Geometry check sheet. Reference: the model listing, model coordinates, mm. Give positions to 0.01 mm unless a question says otherwise; leave off trailing zeros. Write each loop counter-clockwise with the first axis right and the second up, starting at its lowest first coordinate (ties: lowest second). Pieces come first, ordered by that corner, then holes. Notation, with made-up numbers: (-6, -17.75) - (51, -17.75) arc R10 cw to (51, -7.75) - close; hole circle Ø9 at (-15.75, 17). An arc over 180 degrees is marked (long way). Write item = value, one per line. Start each with the question number.
(1) Section check B-B, the plane z = -0.5. Enter the section's corners in (x, y), plus the area to 3 significant figures.
(2) Section check A-A, the plane x = 0. Enter the section's corners in (y, z), plus the area to 3 significant figures.
(3) Thickness scan on L1, parallel to X at y = -7, z = -1.5; L2, parallel to Y at x = -0.25, z = -0.5; L3, parallel to Z at x = 2, y = -6.75. Record the ranges inside material, lowest first.
(4) Section check C-C, the plane z = 10.5. Enter the section's corners in (x, y).
(5) Draft check along X on faces 1 (the cylindrical face through (0.41, -10.123, 28.602)), 2 (the flat face through (0, -4, -11)), 3 (the flat face through (0, -4.35, -5)), 4 (the flat face through (0, -7, 1)). Enter one of: pulls with the +X half, pulls with the -X half, needs draft (parallel to the pull), parting line crosses it, or undercut.
(6) Depth check by flat-ended pin: pin 1 Ø1.8 at (x, y) = (0.5, -7.5) entering from -Z; pin 2 Ø4 at (x, z) = (-1, 25.5) entering from +Y; pin 3 Ø1.5 at (y, z) = (-8.5, 9.5) entering from -X. Enter the tip coordinate at first touch or a pass-through.
```python
from build123d import *

# Parameters (mm, degrees)
BOSS_EXTRUDE1_DEPTH      = 1
BOSS_EXTRUDE1_DEPTH_BACK = 11
BOSS_EXTRUDE2_DEPTH      = 15
SKETCH3_R                = 3.15
BOSS_EXTRUDE3_DEPTH      = 21
FILLET1_R                = 12


with BuildPart() as part:
    # Sketch1 → Boss-Extrude1 (new, two sides: drawn at the far end of the back side and taken through both)
    with BuildSketch(Plane.XY.offset(-BOSS_EXTRUDE1_DEPTH_BACK)):
        with BuildLine():
            Line((2.107130751, -3.6), (-2.107130751, -3.6))
            ThreePointArc((-2.107130751, -3.6), (-3.494890771, -5.054302567), (-4, -7))
            ThreePointArc((-4, -7), (1.945697433, -10.494890771), (2.107130751, -3.6))
        make_face()
        with BuildLine():
            Line((1.881488772, -4.35), (-1.881488772, -4.35))
            ThreePointArc((-1.881488772, -4.35), (-2.887675407, -5.508748598), (-3.25, -7))
            ThreePointArc((-3.25, -7), (1.491251402, -9.887675407), (1.881488772, -4.35))
        make_face(mode=Mode.SUBTRACT)
    extrude(amount=BOSS_EXTRUDE1_DEPTH + BOSS_EXTRUDE1_DEPTH_BACK)

    # Sketch2 → Boss-Extrude2 (add)
    with BuildSketch(Plane.XY.offset(1)):
        with BuildLine():
            Line((2.107130751, -3.6), (-2.107130751, -3.6))
            ThreePointArc((-2.107130751, -3.6), (0, -11), (2.107130751, -3.6))
        make_face()
    extrude(amount=BOSS_EXTRUDE2_DEPTH)

    # Sketch3 → Boss-Extrude3 (add)
    with BuildSketch(Plane.XY.offset(16)):
        with Locations(Location((0, -7, 0), (0, 0, 180))):
            Circle(SKETCH3_R)
    extrude(amount=BOSS_EXTRUDE3_DEPTH)

    # Fillet1
    # the kernel refuses this fillet: 12 mm, written as the material it adds along each edge
    with BuildSketch(Plane(origin=(0, -7, 16), x_dir=(-1, 0, 0), z_dir=(0, 1, 0))) as fillet1_piece_1_section:
        with BuildLine():
            CenterArc((15.15, 4.435932822), FILLET1_R, 180, 21.694716022)
            Line((3.15, 4.435932822), (2.91, 4.435932822))
            Line((2.91, 4.435932822), (2.91, 0))
            Line((2.91, 0), (3.15, -0.24))
            ThreePointArc((3.15, -0.24), (3.575, -0.24), (3.777, -0.088718656))
            Line((3.777, -0.088718656), (4, 0))
        make_face()
    fillet1_piece_1 = revolve(axis=Axis((0, -7, 16), (0, 0, 1)), mode=Mode.PRIVATE)
    fillet1_piece_1 = split(fillet1_piece_1, bisect_by=Plane(origin=(3.32837519, -3.6, 18.170708912), z_dir=(0, -1, 0)), keep=Keep.TOP, mode=Mode.PRIVATE)
    add(fillet1_piece_1)


solid = part.part
```
Model answer:
q1.outline = (-2.11, -3.6) arc R4 ccw (long way) to (2.11, -3.6) - close; hole (-1.88, -4.35) arc R3.25 ccw (long way) to (1.88, -4.35) - close
q1.area = 16.9 mm²
q2.outline = (-11, -11) - (-10.25, -11) - (-10.25, 1) - (-4.35, 1) - (-4.35, -11) - (-3.6, -11) - (-3.6, 18) arc R12 cw to (-3.85, 20.44) - (-3.85, 37) - (-10.15, 37) - (-10.15, 20.44) arc R12 cw to (-11, 16) - close
q2.area = 263 mm²
q3.L1 = -4 to -3.25, 3.25 to 4
q3.L2 = -10.99 to -10.24, -4.35 to -3.6
q3.L3 = 1 to 37
q4.outline = (-2.11, -3.6) arc R4 ccw (long way) to (2.11, -3.6) - close
q5.face_1 = parting line crosses it
q5.face_2 = needs draft
q5.face_3 = undercut
q5.face_4 = undercut
q6.pin_1 = 1
q6.pin_2 = -3.85
q6.pin_3 = -3.93
